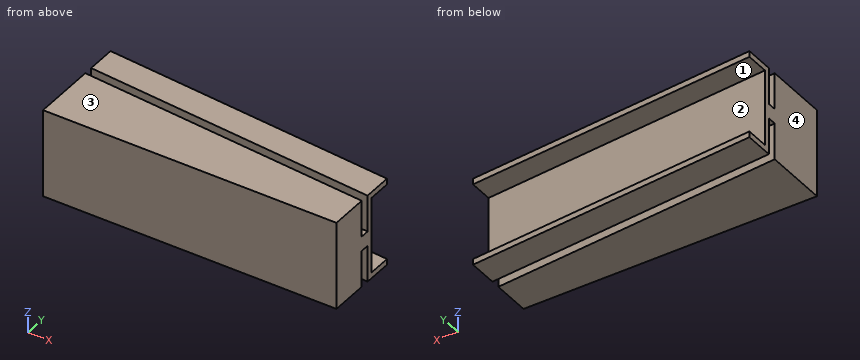
from build123d import *

# Parameters (mm, degrees)
SALIENTE_EXTRUIR1_DEPTH = 30
SALIENTE_EXTRUIR2_DEPTH = 2.5


with BuildPart() as part:
    # Croquis1 → Saliente-Extruir1 (new body)
    with BuildSketch(Plane.XY):
        Polygon((0, 0), (0, 21.748866353), (100, 13), (100, 0), align=None)
    extrude(amount=SALIENTE_EXTRUIR1_DEPTH)

    # Croquis3 → Saliente-Extruir2 (add, symmetric)
    with BuildSketch(Plane.XY.offset(15)):
        Polygon((0, 21.748866353), (100, 13), (100, 16), (0, 24.748866353), align=None)
    extrude(amount=SALIENTE_EXTRUIR2_DEPTH, both=True)

    # Barrer1: sweep along a path in Croquis4
    with BuildLine(Plane.XY.offset(15)) as barrer1_path:
        Line((0, 24.748866353), (100, 16))
    # Croquis5 → Barrer1 (sweep)
    with BuildSketch(Plane.ZY):
        Polygon((28, 34.748866353), (30, 34.748866353), (30, 24.748866353), (0, 24.748866353), (0, 34.748866353), (2, 34.748866353), (2, 26.748866353), (28, 26.748866353), align=None)
    sweep(path=barrer1_path.line)


solid = part.part
Part model, mm, in its own coordinate system. Face numbers are marked on the shaded views. Round coordinates to 2 decimals unless told otherwise and drop trailing zeros. Write each loop counter-clockwise with the first axis right and the second up, starting at its lowest first coordinate (ties: lowest second). Pieces come first, ordered by that corner, then holes. Notation, with made-up numbers: M -34.75,33 L 17.25,33 A10 ccw 17.25,52 Z; hole C 75.5,-27.5 d4. An arc over 180 degrees is marked long. Return JSON: item names as keys, results as strings. Group by question number.
(1) Saw through at B-B on y = 28.5. Write the cut outline in (x, z), then the cut area to 3 significant figures.
(2) Two-plate mould, pull along Z, no slides. Class the marked faces 1, 2, 3 and 4: +Z half, -Z half, draft (parallel to the pull), parting line (faces both ways), or undercut.
(3) Drill centre lines: probe 1 along Z at (x, y) = (45.5, 28.5); probe 2 along Y at (x, z) = (23, 21.25); probe 3 along Y at (x, z) = (90, 18.5). Where is each one in solid material? Low to high.
(4) Saw through at C-C on x = 58. Write the cut outline in (y, z).
(5) Saw through at A-A on z = 4. Write the cut outline in (x, y), then the cut area to 3 significant figures.
(6) Saw through at D-D on z = 13.75. Write the cut outline in (x, y).
(7) Pin check, flat tips, straight feed: pin 1 Ø2 at (y, z) = (15.5, 3.5) entering from -X; pin 2 Ø2 at (x, z) = (56, 4) entering from +Y. Stop position of each tip, or through.
Returned:
{
 "1": {"outline": "M 0,0 L 71.42,0 L 71.42,2 L 0,2 Z; M 0,28 L 71.42,28 L 71.42,30 L 0,30 Z", "area": "286 mm²"},
 "2": {"face 1": "undercut", "face 2": "undercut", "face 3": "+Z half", "face 4": "draft"},
 "3": {"probe 1": "0 to 2, 28 to 30", "probe 2": "0 to 19.74, 22.74 to 24.74", "probe 3": "0 to 13.87, 16.87 to 18.87"},
 "4": {"outline": "M 0,0 L 16.67,0 L 16.67,12.5 L 19.67,12.5 L 19.67,0 L 29.67,0 L 29.67,2 L 21.67,2 L 21.67,28 L 29.67,28 L 29.67,30 L 19.67,30 L 19.67,17.5 L 16.67,17.5 L 16.67,30 L 0,30 Z"},
 "5": {"outline": "M 0,0 L 100,0 L 100,13 L 0,21.75 Z; M 0,24.75 L 100,16 L 100,18 L 0,26.75 Z", "area": "1,940 mm²"},
 "6": {"outline": "M 0,0 L 100,0 L 100,18 L 0,26.75 Z"},
 "7": {"pin 1": "x = 0", "pin 2": "y = 21.94"}
}
